Autodesk Inventor part; units mm, degrees
ref_plane "YZ Plane" through (0, 0, 0) normal (1, 0, 0) x (0, 1, 0)
ref_plane "XZ Plane" through (0, 0, 0) normal (0, 1, 0) x (-1, 0, 0)
ref_plane "XY Plane" through (0, 0, 0) normal (0, 0, 1) x (1, 0, 0)
sketch "Skizze1" plane through (0, 0, 0) normal (0, 1, 0) x (-1, 0, 0)
  line L0 (4.75, -10.5) -> (-4.75, -10.5)
  line L1 (-4.75, -10.5) -> (-4.75, 10.5)
  line L2 (-4.75, 10.5) -> (4.75, 10.5)
  line L3 (4.75, 10.5) -> (4.75, -10.5)
  line L4 (4.75, -10.5) -> (-4.75, 10.5) construction
  line L5 (-4.75, -10.5) -> (4.75, 10.5) construction
  line L6 (-6.75, -12.5) -> (6.75, -12.5)
  line L7 (6.75, -12.5) -> (6.75, 12.5)
  line L8 (6.75, 12.5) -> (-6.75, 12.5)
  line L9 (-6.75, 12.5) -> (-6.75, -12.5)
  line L10 (-6.75, -12.5) -> (6.75, 12.5) construction
  line L11 (6.75, -12.5) -> (-6.75, 12.5) construction
  point P0 (0, 0)
  dimension "d0" = 9.5
  dimension "d1" = 21
  dimension "d2" = 2
  dimension "d3" = 2
extrude "Extrusion1" add sketch "Skizze1" along normal blind 40
sketch "Skizze2" plane through (0, 0, 0) normal (0, -1, 0) x (1, 0, 0)
  line L0 (6.75, 12.5) -> (6.75, -12.5)
  line L1 (-6.75, 12.5) -> (6.75, 12.5)
  line L2 (-6.75, -12.5) -> (-6.75, 12.5)
  line L3 (-6.75, -12.5) -> (6.75, -12.5)
  line L4 (6.75, -12.5) -> (6.75, 12.5)
  line L5 (6.75, 12.5) -> (-6.75, 12.5)
  line L6 (-6.75, 12.5) -> (-6.75, -12.5)
  line L7 (-6.75, -12.5) -> (6.75, 12.5) construction
  line L8 (6.75, -12.5) -> (-6.75, 12.5) construction
  point P0 (0, 0)
extrude "Extrusion2" add sketch "Skizze2" along normal blind 2
sketch "Skizze3" plane through (6.75, 40, -12.5) normal (0, 0, -1) x (-1, 0, 0)
  line L0 (11.5, -40) -> (11.5, 0)
  line L1 (2, -40) -> (2, 0)
  line L2 (11.5, -40) -> (2, -40)
  line L3 (2, -40) -> (2, -37)
  line L4 (2, -37) -> (11.5, -37)
  line L5 (11.5, -37) -> (11.5, -40)
  line L6 (13.5, -42) -> (0, -42)
  line L7 (11.5, -37) -> (13.5, -37)
  line L8 (13.5, -37) -> (13.5, -42)
  line L9 (13.5, -42) -> (11.5, -42)
  line L10 (11.5, -42) -> (11.5, -37)
  line L11 (11.5, -40) -> (11.5, 0)
  line L12 (11.5, -40) -> (5.5, -40)
  line L13 (5.5, -40) -> (5.5, -42)
  line L14 (5.5, -42) -> (11.5, -42)
  line L15 (11.5, -42) -> (11.5, -40)
  point P0 (6.75, -40)
  dimension "d8" = 3
  dimension "d9" = 6
extrude "Extrusion3" cut sketch "Skizze3" against normal up to surface (23 mm away)
chamfer "Fase1" distance 3 angle 45 1 edges at (4.75, 0, -1)
chamfer "Fase2" distance 4 angle 45 1 edges at (6.75, -2, 0)
chamfer "Fase3" distance 4 angle 45 1 edges at (-6.75, -2, 11.5)
fillet "Rundung1" radius 2 2 edges at (4.75, 3, -11.5) (1.25, 0, -1)
fillet "Rundung2" radius 2 1 edges at (4.75, 3, 0)
sketch "Skizze4" plane through (0, 40, 0) normal (0, 1, 0) x (1, 0, 0)
  line L0 (2.75, 12.5) -> (6.75, 12.5)
  line L1 (-6.75, -12.5) -> (6.75, -12.5)
  line L2 (6.75, -12.5) -> (6.75, 12.5)
  line L3 (6.75, 12.5) -> (-6.75, 12.5)
  line L4 (-6.75, 12.5) -> (-6.75, -12.5)
  line L5 (-6.75, -12.5) -> (6.75, 12.5) construction
  line L6 (6.75, -12.5) -> (-6.75, 12.5) construction
  point P0 (0, 0)
extrude "Extrusion4" add sketch "Skizze4" along normal blind 1
equation "\"G_L\" = 0"
equation "\"G_H\" = 0"
equation "\"G_B\" = 0"
properties part number "BackupBat_Wing" material "GEDA Stahl"
Verification items for the finished model (mm, model axes). A direction names the side the tool comes from. Round coordinates to 2 decimals unless told otherwise and drop trailing zeros. Loops run counter-clockwise (first coordinate to the right, second up) from the corner with the lowest first, then second, coordinate; pieces in that order, holes last. Notation, with made-up numbers: (-38.75, 6.5) - (-30.75, 6.5) arc R26 ccw to (-30.75, 21.5) - close; hole circle Ø10 at (40.5, 33). An arc over 180 degrees is marked (long way). Answer in a Markdown table with one row per item. Add a question column.
Q1. Section check A-A on z = 6. Enter the section's corners in (x, y).
Q2. Tool access check on faces 5 (the face through (1.764, 1.975, -11.486)), 6 (the face through (-5, 3, -4)), 7 (the face through (0, 19, 12.5)), 8 (the face through (2.94, 1.19, 0.15)), 9 (the face through (0, 19, 10.5)). Record the directions out of +Z, -Z, +X, -X, +Y, -Y that give a thin tool (end or side, any length) a straight path to the whole face; none if there is none.
Q3. Section check C-C on x = -3.5. Enter the section's corners in (y, z).
Q4. Release check for a two-part mould opening along Y. For faces 1 (the face through (0, 40, 0)), 2 (the face through (0, 41, 0)), 3 (the face through (-4.78, 0.03, 11.51)), 4 (the face through (-4.75, 21, 0)) record: pulls with the +Y half, pulls with the -Y half, needs draft (parallel to the pull), parting line crosses it, or undercut.
Q5. Section check D-D on x = 0.75. Enter the section's corners in (y, z).
Q6. Gauge pin test, flat ends, axial feed: pin 1 (3 mm diameter, centred on x = -3.5, z = -2, fed in from -Y); pin 2 (2 mm diameter, centred on x = 0, z = 5, fed in from -Y). Record the tip position at first contact, or that the pin passes through.
Q7. Section check B-B on y = 36. Enter the section's corners in (x, z), plus the area to 3 significant figures.
Q8. Material ranges on line 1 (Z direction, x = -3.5, y = 8.5); line 2 (X direction, y = 25, z = -10); line 3 (Y direction, x = -3, z = 7.5), recorded low to high.
Found:
| question | item | result |
|---|---|---|
| 1 | outline | (-6.75, 3) - (-4.75, 3) - (-4.75, 40) - (4.75, 40) - (4.75, 3.83) arc R2 cw to (4.16, 2.41) - (1.75, 0) arc R2 ccw to (1.25, -1.32) - (1.25, -2) - (2.75, -2) - (6.75, 2) - (6.75, 41) - (-6.75, 41) - close |
| 2 | face 5 | -Z, -X |
| 2 | face 6 | -Z, -X, -Y |
| 2 | face 7 | +Z, +X, -X, +Y, -Y |
| 2 | face 8 | -X |
| 2 | face 9 | none |
| 3 | outline | (-1.25, 10.5) - (40, 10.5) - (40, -10.5) - (3, -10.5) - (3, -12.5) - (41, -12.5) - (41, 12.5) - (-1.25, 12.5) - close |
| 4 | face 1 | undercut |
| 4 | face 2 | pulls with the +Y half |
| 4 | face 3 | pulls with the -Y half |
| 4 | face 4 | needs draft |
| 5 | outline | (-2, 10.5) - (40, 10.5) - (40, -10.5) - (2.86, -10.5) - (2.86, -12.5) - (41, -12.5) - (41, 12.5) - (-2, 12.5) - close |
| 6 | pin 1 | stops at y = 3 |
| 6 | pin 2 | stops at y = 40 |
| 7 | outline | (-6.75, -12.5) - (6.75, -12.5) - (6.75, 12.5) - (-6.75, 12.5) - close; hole (-4.75, -10.5) - (4.75, -10.5) - (4.75, 10.5) - (-4.75, 10.5) - close |
| 7 | area | 138 mm² |
| 8 | line 1 | z = -12.5 to -10.5, 10.5 to 12.5 |
| 8 | line 2 | x = -6.75 to -4.75, 4.75 to 6.75 |
| 8 | line 3 | y = 40 to 41 |
